from build123d import *

# Parameters (mm, degrees)
SM_BASE_FLANGE_3_DEPTH        = 3
SM_EDGE_FLANGE_6_DEPTH        = 200
SM_EDGE_FLANGE_6_BEND_DEPTH   = 200
SM_EDGE_FLANGE_6_BEND_2_DEPTH = 200
CUT_EXTRUDE_4_REACH           = 325.007
SKETCH_47_R                   = 2
CUT_EXTRUDE_6_REACH           = 239.77
SKETCH_50_R                   = 2
CUT_EXTRUDE_7_REACH           = 313.862
SKETCH_51_R                   = 2
CUT_EXTRUDE_8_REACH           = 310.931
SKETCH_52_R                   = 13.5


# Sheet-metal steps are written as plain solids
with BuildPart() as part:
    # Эскиз10 → Базовая кромка3 (new body)
    with BuildSketch(Plane.XY):
        Polygon((0, 0), (-21, 36.373066959), (79, 209.578147716), (121, 209.578147716), (221, 36.373066959), (200, 0), align=None)
    extrude(amount=-SM_BASE_FLANGE_3_DEPTH)

    # Ребро-кромка6 section (across the edge) → Ребро-кромка6 (add)
    with BuildSketch(Plane(origin=(-21.866025404, 36.873066959, -3), x_dir=(0.8660254037844437, -0.4999999999999915, -3.4914813388431334e-15), z_dir=(0.4999999999999915, 0.8660254037844437, 0))):
        with BuildLine():
            Line((-3, 1), (-3, 17))
            Line((-3, 17), (0, 17))
            Line((0, 17), (0, 1))
            ThreePointArc((0, 1), (0.292893219, 0.292893219), (1, 0))
            Line((1, 0), (1, -3))
            ThreePointArc((1, -3), (-1.828427125, -1.828427125), (-3, 1))
        make_face()
    extrude(amount=SM_EDGE_FLANGE_6_DEPTH)

    # Ребро-кромка6 section 2 (across the edge) → Ребро-кромка6 bend (add)
    with BuildSketch(Plane(origin=(121.866025404, 210.078147716, -3), x_dir=(-0.8660254037844362, -0.5000000000000044, -3.491481338843134e-15), z_dir=(0.5000000000000044, -0.8660254037844362, 0))):
        with BuildLine():
            Line((-3, 1), (-3, 17))
            Line((-3, 17), (0, 17))
            Line((0, 17), (0, 1))
            ThreePointArc((0, 1), (0.292893219, 0.292893219), (1, 0))
            Line((1, 0), (1, -3))
            ThreePointArc((1, -3), (-1.828427125, -1.828427125), (-3, 1))
        make_face()
    extrude(amount=SM_EDGE_FLANGE_6_BEND_DEPTH)

    # Ребро-кромка6 section 3 (across the edge) → Ребро-кромка6 bend 2 (add)
    with BuildSketch(Plane(origin=(200, -1, -3), x_dir=(0, 1, 0), z_dir=(-1, 0, 0))):
        with BuildLine():
            Line((-3, 1), (-3, 17))
            Line((-3, 17), (0, 17))
            Line((0, 17), (0, 1))
            ThreePointArc((0, 1), (0.292893219, 0.292893219), (1, 0))
            Line((1, 0), (1, -3))
            ThreePointArc((1, -3), (-1.828427125, -1.828427125), (-3, 1))
        make_face()
    extrude(amount=SM_EDGE_FLANGE_6_BEND_2_DEPTH)

    # Эскиз47 → Вырез-Вытянуть4 (cut, up to next)
    with BuildSketch(Plane(origin=(-34.964101615, 20.186533479, 0), x_dir=(0, 0, 1), z_dir=(-0.866025403784443, 0.4999999999999925, 3.788649256556814e-15)), mode=Mode.PRIVATE) as cut_extrude_4_sk1:
        with Locations(Location((-12, 29, 0), (0, 0, 270))):
            Circle(SKETCH_47_R)
    cut_extrude_4_tool1 = extrude(cut_extrude_4_sk1.sketch, amount=-CUT_EXTRUDE_4_REACH, mode=Mode.PRIVATE) & part.part
    # Эскиз47 → Вырез-Вытянуть4 (cut, up to next)
    with BuildSketch(Plane(origin=(-34.964101615, 20.186533479, 0), x_dir=(0, 0, 1), z_dir=(-0.866025403784443, 0.4999999999999925, 3.788649256556814e-15)), mode=Mode.PRIVATE) as cut_extrude_4_sk2:
        with Locations(Location((-12, 39, 0), (0, 0, 270))):
            Circle(SKETCH_47_R)
    cut_extrude_4_tool2 = extrude(cut_extrude_4_sk2.sketch, amount=-CUT_EXTRUDE_4_REACH, mode=Mode.PRIVATE) & part.part
    # Эскиз47 → Вырез-Вытянуть4 (cut, up to next)
    with BuildSketch(Plane(origin=(-34.964101615, 20.186533479, 0), x_dir=(0, 0, 1), z_dir=(-0.866025403784443, 0.4999999999999925, 3.788649256556814e-15)), mode=Mode.PRIVATE) as cut_extrude_4_sk3:
        with Locations(Location((-12, 203, 0), (0, 0, 270))):
            Circle(SKETCH_47_R)
    cut_extrude_4_tool3 = extrude(cut_extrude_4_sk3.sketch, amount=-CUT_EXTRUDE_4_REACH, mode=Mode.PRIVATE) & part.part
    # Эскиз47 → Вырез-Вытянуть4 (cut, up to next)
    with BuildSketch(Plane(origin=(-34.964101615, 20.186533479, 0), x_dir=(0, 0, 1), z_dir=(-0.866025403784443, 0.4999999999999925, 3.788649256556814e-15)), mode=Mode.PRIVATE) as cut_extrude_4_sk4:
        with Locations(Location((-12, 213, 0), (0, 0, 270))):
            Circle(SKETCH_47_R)
    cut_extrude_4_tool4 = extrude(cut_extrude_4_sk4.sketch, amount=-CUT_EXTRUDE_4_REACH, mode=Mode.PRIVATE) & part.part
    add(cut_extrude_4_tool1.solids().sort_by_distance((-20.464102, 45.30127, -12))[0], mode=Mode.SUBTRACT)
    add(cut_extrude_4_tool2.solids().sort_by_distance((-15.464102, 53.961524, -12))[0], mode=Mode.SUBTRACT)
    add(cut_extrude_4_tool3.solids().sort_by_distance((66.535898, 195.98969, -12))[0], mode=Mode.SUBTRACT)
    add(cut_extrude_4_tool4.solids().sort_by_distance((71.535898, 204.649944, -12))[0], mode=Mode.SUBTRACT)

    # Эскиз50 → Вырез-Вытянуть6 (cut, up to next)
    with BuildSketch(Plane(origin=(184.964101615, 106.789073858, 0), x_dir=(0, 0, -1), z_dir=(0.866025403784436, 0.5000000000000047, 3.0623287353932815e-15)), mode=Mode.PRIVATE) as cut_extrude_6_sk1:
        with Locations(Location((12, -71, 0), (0, 0, 90))):
            Circle(SKETCH_50_R)
    cut_extrude_6_tool1 = extrude(cut_extrude_6_sk1.sketch, amount=-CUT_EXTRUDE_6_REACH, mode=Mode.PRIVATE) & part.part
    # Эскиз50 → Вырез-Вытянуть6 (cut, up to next)
    with BuildSketch(Plane(origin=(184.964101615, 106.789073858, 0), x_dir=(0, 0, -1), z_dir=(0.866025403784436, 0.5000000000000047, 3.0623287353932815e-15)), mode=Mode.PRIVATE) as cut_extrude_6_sk2:
        with Locations(Location((12, -61, 0), (0, 0, 90))):
            Circle(SKETCH_50_R)
    cut_extrude_6_tool2 = extrude(cut_extrude_6_sk2.sketch, amount=-CUT_EXTRUDE_6_REACH, mode=Mode.PRIVATE) & part.part
    # Эскиз50 → Вырез-Вытянуть6 (cut, up to next)
    with BuildSketch(Plane(origin=(184.964101615, 106.789073858, 0), x_dir=(0, 0, -1), z_dir=(0.866025403784436, 0.5000000000000047, 3.0623287353932815e-15)), mode=Mode.PRIVATE) as cut_extrude_6_sk3:
        with Locations(Location((12, 103, 0), (0, 0, 90))):
            Circle(SKETCH_50_R)
    cut_extrude_6_tool3 = extrude(cut_extrude_6_sk3.sketch, amount=-CUT_EXTRUDE_6_REACH, mode=Mode.PRIVATE) & part.part
    # Эскиз50 → Вырез-Вытянуть6 (cut, up to next)
    with BuildSketch(Plane(origin=(184.964101615, 106.789073858, 0), x_dir=(0, 0, -1), z_dir=(0.866025403784436, 0.5000000000000047, 3.0623287353932815e-15)), mode=Mode.PRIVATE) as cut_extrude_6_sk4:
        with Locations(Location((12, 113, 0), (0, 0, 90))):
            Circle(SKETCH_50_R)
    cut_extrude_6_tool4 = extrude(cut_extrude_6_sk4.sketch, amount=-CUT_EXTRUDE_6_REACH, mode=Mode.PRIVATE) & part.part
    add(cut_extrude_6_tool1.solids().sort_by_distance((220.464102, 45.30127, -12))[0], mode=Mode.SUBTRACT)
    add(cut_extrude_6_tool2.solids().sort_by_distance((215.464102, 53.961524, -12))[0], mode=Mode.SUBTRACT)
    add(cut_extrude_6_tool3.solids().sort_by_distance((133.464102, 195.98969, -12))[0], mode=Mode.SUBTRACT)
    add(cut_extrude_6_tool4.solids().sort_by_distance((128.464102, 204.649944, -12))[0], mode=Mode.SUBTRACT)

    # Эскиз51 → Вырез-Вытянуть7 (cut, up to next)
    with BuildSketch(Plane.XZ.offset(4), mode=Mode.PRIVATE) as cut_extrude_7_sk1:
        with Locations(Location((192, -12, 0), (0, 0, 270))):
            Circle(SKETCH_51_R)
    cut_extrude_7_tool1 = extrude(cut_extrude_7_sk1.sketch, amount=-CUT_EXTRUDE_7_REACH, mode=Mode.PRIVATE) & part.part
    # Эскиз51 → Вырез-Вытянуть7 (cut, up to next)
    with BuildSketch(Plane.XZ.offset(4), mode=Mode.PRIVATE) as cut_extrude_7_sk2:
        with Locations(Location((182, -12, 0), (0, 0, 270))):
            Circle(SKETCH_51_R)
    cut_extrude_7_tool2 = extrude(cut_extrude_7_sk2.sketch, amount=-CUT_EXTRUDE_7_REACH, mode=Mode.PRIVATE) & part.part
    # Эскиз51 → Вырез-Вытянуть7 (cut, up to next)
    with BuildSketch(Plane.XZ.offset(4), mode=Mode.PRIVATE) as cut_extrude_7_sk3:
        with Locations(Location((18, -12, 0), (0, 0, 270))):
            Circle(SKETCH_51_R)
    cut_extrude_7_tool3 = extrude(cut_extrude_7_sk3.sketch, amount=-CUT_EXTRUDE_7_REACH, mode=Mode.PRIVATE) & part.part
    # Эскиз51 → Вырез-Вытянуть7 (cut, up to next)
    with BuildSketch(Plane.XZ.offset(4), mode=Mode.PRIVATE) as cut_extrude_7_sk4:
        with Locations(Location((8, -12, 0), (0, 0, 270))):
            Circle(SKETCH_51_R)
    cut_extrude_7_tool4 = extrude(cut_extrude_7_sk4.sketch, amount=-CUT_EXTRUDE_7_REACH, mode=Mode.PRIVATE) & part.part
    add(cut_extrude_7_tool1.solids().sort_by_distance((192, -4, -12))[0], mode=Mode.SUBTRACT)
    add(cut_extrude_7_tool2.solids().sort_by_distance((182, -4, -12))[0], mode=Mode.SUBTRACT)
    add(cut_extrude_7_tool3.solids().sort_by_distance((18, -4, -12))[0], mode=Mode.SUBTRACT)
    add(cut_extrude_7_tool4.solids().sort_by_distance((8, -4, -12))[0], mode=Mode.SUBTRACT)

    # Эскиз52 → Вырез-Вытянуть8 (cut, up to next)
    with BuildSketch(Plane(origin=(0, 0, -3), x_dir=(-1, 0, 0), z_dir=(0, 0, -1)), mode=Mode.PRIVATE) as cut_extrude_8_sk1:
        with Locations((-100, 81.983738225)):
            Circle(SKETCH_52_R)
    cut_extrude_8_tool1 = extrude(cut_extrude_8_sk1.sketch, amount=-CUT_EXTRUDE_8_REACH, mode=Mode.PRIVATE) & part.part
    add(cut_extrude_8_tool1.solids().sort_by_distance((100, 81.983738, -3))[0], mode=Mode.SUBTRACT)


solid = part.part
Here's how the part is built. I have some questions about the finished solid (model axes, mm). A direction names the side the tool comes from. Give positions to 0.01 mm unless a question says otherwise; leave off trailing zeros. Loops run counter-clockwise (first coordinate to the right, second up) from the corner with the lowest first, then second, coordinate; pieces in that order, holes last. Notation, with made-up numbers: (-19, -24.75) -> (40, -24.75) arc R23 cw to (40, 4.25) -> close; hole circle Ø8 at (12, -35.75). An arc over 180 degrees is marked (long way). Answer as a JSON object with one key per item and string values. Group by question number.
Item 1: Thinking about a two-plate mould opening in Y: for faces 4 (the cylindrical face through (27.68, 122.12, -3.3)), 5 (the flat face through (173.764, 126.188, -11.888)), 6 (the flat face through (101, -4, -12)), 7 (the flat face through (75, 83, 0)), which applies, pulls with the +Y half, pulls with the -Y half, needs draft (parallel to the pull), parting line crosses it, or undercut?
Item 2: Imagine slicing it at B-B on x = 100. Write out the boundary of the cut face in (y, z).
Item 3: On a 3-axis mill with a long thin cutter (end or side, diameter ignored), from which of +Z, -Z, +X, -X, +Y, -Y can I reach the whole of each face in a straight line? I mean faces 1 (the flat face through (171.166, 124.688, -12.112)), 2 (the flat face through (101, -1, -12)), 3 (the cylindrical face through (25.88, 123.16, -1.14)). Say none if no direction works.
Item 4: I need wall thicknesses on L1, parallel to X at y = -3.1, z = -12; L2, parallel to Y at x = 196, z = -15; L3, parallel to Y at x = 64, z = -10. Which ranges of each line are inside material? Lowest first, please.
Item 5: Imagine slicing it at A-A on z = -17.25. Write out the boundary of the cut face in (x, y), then the cut area to 3 significant figures.
Item 6: Will these pins go through, and if not, where does the flat tip stop? pin 1 (3 mm diameter, centred on y = 127.5, z = -7, fed in from -X); pin 2 (8 mm diameter, centred on x = 130, z = -11, fed in from +Y); pin 3 (3.5 mm diameter, centred on x = 8, z = -12, fed in from -Y).
Answer list:
{
 "1": {"face 4": "undercut", "face 5": "pulls with the +Y half", "face 6": "pulls with the -Y half", "face 7": "needs draft"},
 "2": {"outline": "(-4, -20) -> (-1, -20) -> (-1, -4) arc R1 cw to (0, -3) -> (68.48, -3) -> (68.48, 0) -> (0, 0) arc R4 ccw to (-4, -4) -> close; (95.48, -3) -> (209.58, -3) -> (209.58, 0) -> (95.48, 0) -> close"},
 "3": {"face 1": "-Z", "face 2": "-Z, +X, -X", "face 3": "+Z, -X, +Y"},
 "4": {"L1": "x = 0 to 6, 10 to 16, 20 to 180, 184 to 190, 194 to 200", "L2": "y = -4 to -1, 81.67 to 87.67", "L3": "y = -4 to -1, 185.6 to 191.6"},
 "5": {"outline": "(-24.46, 38.37) -> (-21.87, 36.87) -> (78.13, 210.08) -> (75.54, 211.58) -> close; (0, -4) -> (200, -4) -> (200, -1) -> (0, -1) -> close; (121.87, 210.08) -> (221.87, 36.87) -> (224.46, 38.37) -> (124.46, 211.58) -> close", "area": "1,800 mm2"},
 "6": {"pin 1": "stops at x = 26.13", "pin 2": "stops at y = 208.92", "pin 3": "stops at y = 85.57"}
}
